```python
from build123d import *

# Parameters (mm, degrees)
F0_W     = 7.2136
F0_H     = 10.287
F0_H_2   = 17.4625
F0_W_2   = 15.0114
F2_R     = 1.5875
F3_SIZE  = 0.79375
F4_SIZE2 = 6.35
F4_SIZE  = 1.5748


with BuildPart() as f1:
    # F0 (on Right) → F1 (revolve)
    with BuildSketch(Plane.YZ):
        with Locations((3.6068, 30.5435)):
            Rectangle(F0_W, F0_H)
        with Locations((3.6068, 16.66875)):
            Rectangle(F0_W, F0_H_2)
        with Locations((14.7193, 16.66875)):
            Rectangle(F0_W_2, F0_H_2)
    revolve(axis=Axis((0, 6.4671109096, 0), (0, 1, 0)))

    # F2
    f2_edges = [f1.edges().sort_by_distance(p)[0] for p in [
        (0, 7.2136, -35.687),
    ]]
    fillet(f2_edges, radius=F2_R)

    # F3
    f3_edges = [f1.edges().sort_by_distance(p)[0] for p in [
        (0, 22.225, -25.4),
    ]]
    chamfer(f3_edges, length=F3_SIZE)

    # F4
    f4_edges = [f1.edges().sort_by_distance(p)[0] for p in [
        (0, 0, -35.687),
        (0, 5.6261, -35.687),
    ]]
    f4_side = f1.faces().sort_by_distance((0, 2.81305, -35.687))[0]
    chamfer(f4_edges, length=F4_SIZE, length2=F4_SIZE2, reference=f4_side)


solid = f1.part
```
Check sheet for the modelled part. Datum: model origin and axes. Units: mm. A direction names the side the tool comes from. Round coordinates to 2 decimals unless told otherwise and drop trailing zeros. Order: outer loops, then holes, each group sorted by start corner. A loop starts at its lowest first (then second) coordinate and runs counter-clockwise, first axis right, second up. Notation, with made-up numbers: M 37.5,51 L 72.5,51 A30 cw 72.5,73 Z; hole C 64.5,59.25 d1. An arc over 180 degrees is marked long. Answer in a Markdown table with one row per item.
(1) Section check A-A on x = 0. Record the boundary of the cut face in (y, z) (1 decimal), plus the area to 3 significant figures.
Findings:
| item | result |
|---|---|
| outline | M 0,-29.3 L 1.6,-35.7 L 5.6,-35.7 A1.6 ccw 7.2,-34.1 L 7.2,-25.4 L 21.4,-25.4 L 22.2,-24.6 L 22.2,-7.9 L 0,-7.9 Z; M 0,7.9 L 22.2,7.9 L 22.2,24.6 L 21.4,25.4 L 7.2,25.4 L 7.2,34.1 A1.6 ccw 5.6,35.7 L 1.6,35.7 L 0,29.3 Z |
| area | 913 mm^2 |
(2) Section check D-D on y = 3.5. Record the boundary of the cut face in (x, z) (1 decimal), plus the area to 3 significant figures.
Findings:
| item | result |
|---|---|
| outline | C 0,0 d71.4; hole C 0,0 d15.9 |
| area | 3,800 mm^2 |
(3) Draft check along X on faces 3 (the flat face through (25.4, 7.214, 5.2)), 4 (the cylindrical face through (-7.75, 11.27, -1.72)), 5 (the conical face through (-28.94, 0.076, -6.427)). Enter one of: +X half, -X half, draft (parallel to the pull), parting line (faces both ways), or undercut.
Findings:
| item | result |
|---|---|
| face 3 | draft |
| face 4 | undercut |
| face 5 | parting line |
(4) Section check B-B on z = 0. Record the boundary of the cut face in (x, y) (1 decimal), plus the area to 3 significant figures.
Findings:
| item | result |
|---|---|
| outline | M -35.7,1.6 L -29.3,0 L -7.9,0 L -7.9,22.2 L -24.6,22.2 L -25.4,21.4 L -25.4,7.2 L -34.1,7.2 A1.6 ccw -35.7,5.6 Z; M 7.9,0 L 29.3,0 L 35.7,1.6 L 35.7,5.6 A1.6 ccw 34.1,7.2 L 25.4,7.2 L 25.4,21.4 L 24.6,22.2 L 7.9,22.2 Z |
| area | 913 mm^2 |
(5) Material ranges on line 1 along X through (y, z) = (17, 0); line 2 along X through (y, z) = (5, 0); line 3 along Y through (x, z) = (-7, -25), recorded low to high. Write a range as from..to.
Findings:
| item | result |
|---|---|
| line 1 | x = -25.4..-7.94, 7.94..25.4 |
| line 2 | x = -35.69..-7.94, 7.94..35.69 |
| line 3 | y = 0..7.21 |
(6) Section check C-C on y = 11.5. Record the boundary of the cut face in (x, z) (1 decimal), plus the area to 3 significant figures.
Findings:
| item | result |
|---|---|
| outline | C 0,0 d50.8; hole C 0,0 d15.9 |
| area | 1,830 mm^2 |
(7) Gauge pin test, flat ends, axial feed: pin 1 (6 mm diameter, centred on x = 15.5, y = 15, fed in from +Z); pin 2 (2 mm diameter, centred on x = 15, y = 4, fed in from +Z); pin 3 (10 mm diameter, centred on y = 10.5, z = 10.5, fed in from -X). Record the tip position at first contact, or that the pin passes through.
Findings:
| item | result |
|---|---|
| pin 1 | stops at z = 22.11 |
| pin 2 | stops at z = 32.83 |
| pin 3 | stops at x = -34.68 |
(8) Set-up check for faces 1 (the flat face through (-6, 0, 6)), 2 (the cylindrical face through (-24.796, 14.422, -5.506)): record each of +Z, -Z, +X, -X, +Y, -Y from which the full face is reachable in a straight line by a thin tool's end or side.
Findings:
| item | result |
|---|---|
| face 1 | +Z, -Z, +X, -X, -Y |
| face 2 | +Y |
